Check sheet for the modelled part. Datum: model origin and axes. Units: mm. A direction names the side the tool comes from. Give positions to 0.01 mm unless a question says otherwise; leave off trailing zeros. Write each loop counter-clockwise with the first axis right and the second up, starting at its lowest first coordinate (ties: lowest second). Pieces come first, ordered by that corner, then holes. Notation, with made-up numbers: (-40, 24.25) -> (-33, 24.25) arc R24 ccw to (-33, 35.25) -> close; hole circle Ø2 at (2.25, 80). An arc over 180 degrees is marked (long way). Answer as a JSON object with one key per item and string values.
from build123d import *

# Parameters (mm, degrees)
F0_W     = 40.9
F0_H     = 10
F0_H_2   = 5
F1_DEPTH = 26.8
F2_DEPTH = 2.5


with BuildPart() as f1:
    # F0 (on Top) → F1 (new body)
    with BuildSketch(Plane.XY):
        Rectangle(F0_W, F0_H)
        with Locations((0, -7.5)):
            Rectangle(F0_W, F0_H_2)
        with Locations((0, 7.5)):
            Rectangle(F0_W, F0_H_2)
    extrude(amount=-F1_DEPTH)

    # F0 (on Top) → F2 (join)
    with BuildSketch(Plane.XY):
        with BuildLine():
            Line((-21.25, 5), (-20.45, 5))
            Line((-20.45, 5), (-20.45, 10))
            Line((-20.45, 10), (-25, 10))
            ThreePointArc((-25, 10), (-26.4142135624, 9.4142135624), (-27, 8))
            Line((-27, 8), (-27, 6.1989578808))
            ThreePointArc((-27, 6.1989578808), (-23.6376275643, 7.9368350311), (-21.25, 5))
        make_face()
        with BuildLine():
            Line((-21.25, -5), (-20.45, -5))
            Line((-20.45, -5), (-20.45, 5))
            Line((-20.45, 5), (-21.25, 5))
            ThreePointArc((-21.25, 5), (-22.1286796564, 2.8786796564), (-24.25, 2))
            Line((-24.25, 2), (-24.25, -2))
            ThreePointArc((-24.25, -2), (-22.1286796564, -2.8786796564), (-21.25, -5))
        make_face()
        with BuildLine():
            ThreePointArc((-27, -3.8010421192), (-25.8936432638, -2.4903313324), (-24.25, -2))
            Line((-24.25, -2), (-24.25, 2))
            ThreePointArc((-24.25, 2), (-25.8936432638, 2.4903313324), (-27, 3.8010421192))
            Line((-27, 3.8010421192), (-27, -3.8010421192))
        make_face()
        with BuildLine():
            Line((-25, -10), (-20.45, -10))
            Line((-20.45, -10), (-20.45, -5))
            Line((-20.45, -5), (-21.25, -5))
            ThreePointArc((-21.25, -5), (-23.6376275643, -7.9368350311), (-27, -6.1989578808))
            Line((-27, -6.1989578808), (-27, -8))
            ThreePointArc((-27, -8), (-26.4142135624, -9.4142135624), (-25, -10))
        make_face()
        with Locations((0, -7.5)):
            Rectangle(F0_W, F0_H_2)
        Rectangle(F0_W, F0_H)
        with BuildLine():
            Line((20.45, -5), (20.45, -10))
            Line((20.45, -10), (25, -10))
            ThreePointArc((25, -10), (26.4142135624, -9.4142135624), (27, -8))
            Line((27, -8), (27, -6.1989578808))
            ThreePointArc((27, -6.1989578808), (23.6376275643, -7.9368350311), (21.25, -5))
            Line((21.25, -5), (20.45, -5))
        make_face()
        with Locations((0, 7.5)):
            Rectangle(F0_W, F0_H_2)
        with BuildLine():
            Line((20.45, 10), (20.45, 5))
            Line((20.45, 5), (21.25, 5))
            ThreePointArc((21.25, 5), (23.6376275643, 7.9368350311), (27, 6.1989578808))
            Line((27, 6.1989578808), (27, 8))
            ThreePointArc((27, 8), (26.4142135624, 9.4142135624), (25, 10))
            Line((25, 10), (20.45, 10))
        make_face()
        with BuildLine():
            Line((20.45, 5), (20.45, -5))
            Line((20.45, -5), (21.25, -5))
            ThreePointArc((21.25, -5), (22.1286796564, -2.8786796564), (24.25, -2))
            Line((24.25, -2), (24.25, 2))
            ThreePointArc((24.25, 2), (22.1286796564, 2.8786796564), (21.25, 5))
            Line((21.25, 5), (20.45, 5))
        make_face()
        with BuildLine():
            Line((24.25, 2), (24.25, -2))
            ThreePointArc((24.25, -2), (25.8936432638, -2.4903313324), (27, -3.8010421192))
            Line((27, -3.8010421192), (27, 3.8010421192))
            ThreePointArc((27, 3.8010421192), (25.8936432638, 2.4903313324), (24.25, 2))
        make_face()
    extrude(amount=F2_DEPTH)


solid = f1.part
1. Scan line: L1, parallel to X at y = 9, z = -4. Record every from-to range of solid material in increasing order. Write a range as [from, to].
Determined:
{"L1": "[-20.45, 20.45]"}
2. Go/stop test with flat-tipped pins: P1, Ø2, axis at x = -22.5, y = 3, coming from the -Z side; P2, Ø12, axis at y = 2, z = -12, coming from the -X side; P3, Ø10, axis at y = -1.5, z = -8.5, coming from the +X side. Record where each tip stops, or that it passes through.
Determined:
{"P1": "z = 0", "P2": "x = -20.45", "P3": "x = 20.45"}
3. Sectioned sample at C-C, the plane z = -2. Enter the section's corners in (x, y), plus the area to 3 significant figures.
Determined:
{"outline": "(-20.45, -10) -> (20.45, -10) -> (20.45, 10) -> (-20.45, 10) -> close", "area": "818 mm^2"}
4. Access from +Z, -Z, +X, -X, +Y, -Y to the whole of each face (thin tool, end or side, straight path). Record for faces 1 (the face through (-26.4, 9.43, 1.23)), 2 (the face through (-20.45, 0, -13)), 3 (the face through (23, 0, 0)).
Determined:
{"face 1": "+Z, -Z, -X, +Y", "face 2": "-Z, -X, +Y, -Y", "face 3": "-Z, +X, +Y, -Y"}
5. Sectioned sample at A-A, the plane y = 6.75. Enter the section's corners in (x, z), plus the area to 3 significant figures.
Determined:
{"outline": "(-27, 0) -> (-26.69, 0) -> (-26.69, 2.5) -> (-27, 2.5) -> close; (-21.81, 0) -> (-20.45, 0) -> (-20.45, -26.8) -> (20.45, -26.8) -> (20.45, 0) -> (21.81, 0) -> (21.81, 2.5) -> (-21.81, 2.5) -> close; (26.69, 0) -> (27, 0) -> (27, 2.5) -> (26.69, 2.5) -> close", "area": "1,210 mm^2"}
6. Sectioned sample at B-B, the plane x = -23.5. Enter the section's corners in (y, z), plus the area to 3 significant figures.
Determined:
{"outline": "(-10, 0) -> (-7.9, 0) -> (-7.9, 2.5) -> (-10, 2.5) -> close; (-2.1, 0) -> (2.1, 0) -> (2.1, 2.5) -> (-2.1, 2.5) -> close; (7.9, 0) -> (10, 0) -> (10, 2.5) -> (7.9, 2.5) -> close", "area": "21.0 mm^2"}
